Input: part model. Units: mm. Frame: model coordinates. A direction names the side the tool comes from. Round coordinates to 2 decimals unless told otherwise and drop trailing zeros. Write each loop counter-clockwise with the first axis right and the second up, starting at its lowest first coordinate (ties: lowest second). Pieces come first, ordered by that corner, then holes. Notation, with made-up numbers: (66.25, 17) -> (93.25, 17) arc R11 ccw to (93.25, 31) -> close; hole circle Ø8 at (-4.5, -9). An arc over 180 degrees is marked (long way). Write item = value, one per line.
```python
from build123d import *

# Parameters (mm, degrees)
SKETCH1_R               = 5.5
BOSS_EXTRUDE1_DEPTH     = 23
SKETCH2_R               = 4.5
BOSS_EXTRUDE2_DEPTH     = 6
SKETCH3_R               = 1.5
CUT_EXTRUDE1_DEPTH      = 6.5
CUT_EXTRUDE1_DEPTH_BACK = 6.5


with BuildPart() as part:
    # Sketch1 → Boss-Extrude1 (new body)
    with BuildSketch(Plane.XY):
        Circle(SKETCH1_R)
    extrude(amount=BOSS_EXTRUDE1_DEPTH)

    # Sketch2 → Boss-Extrude2 (add)
    with BuildSketch(Plane.XY.offset(23)):
        Circle(SKETCH2_R)
    extrude(amount=BOSS_EXTRUDE2_DEPTH)

    # Sketch3 → Cut-Extrude1 (cut, two sides)
    with BuildSketch(Plane(origin=(0, 0, 0), x_dir=(1, 0, 0), z_dir=(0, 1, 0))) as cut_extrude1_sk:
        with Locations((0, -26)):
            Circle(SKETCH3_R)
    extrude(amount=CUT_EXTRUDE1_DEPTH, mode=Mode.SUBTRACT)
    extrude(cut_extrude1_sk.sketch, amount=-CUT_EXTRUDE1_DEPTH_BACK, mode=Mode.SUBTRACT)


solid = part.part
```
1) Cut plane B-B (y = 2.5). Return the cut outline in (x, z), and give its area (3 significant figures).
Solutions:
outline = (-4.9, 0) -> (4.9, 0) -> (4.9, 23) -> (3.74, 23) -> (3.74, 29) -> (-3.74, 29) -> (-3.74, 23) -> (-4.9, 23) -> close; hole circle Ø3 at (0, 26)
area = 263 mm^2
2) Access query for faces 1 (the face through (-1.19, -5.37, 11.34)), 2 (the face through (-5, 0, 23)). Directions: +Z, -Z, +X, -X, +Y, -Y. A direction counts if a zero-diameter tool reaches every point of the face in a straight line with its end or side. Return the directions, or none.
Solutions:
face_1 = +Z, -Z
face_2 = +Z
3) Cut plane D-D (z = 6.5). Return the cut outline in (x, y).
Solutions:
outline = circle Ø11 at (0, 0)
4) First-contact query: P1, Ø3.5, axis at x = 0, z = 26, coming from the +Y side; P2, Ø5, axis at x = 0, z = 26, coming from the -Y side; P3, Ø4, axis at y = -4, z = 3, coming from the +X side. Flat tips, straight axial feed; report the tip coordinate or a pass-through.
Solutions:
P1 = 4.5
P2 = -4.5
P3 = 5.12
5) Line query: L1, parallel to Z at x = 0, y = 1.5; L2, parallel to Z at x = -0.5, y = 0; L3, parallel to X at y = 1.9, z = 26. Output: solid intervals per line, ascending. Write a range as from..to.
Solutions:
L1 = 0..24.5, 27.5..29
L2 = 0..24.59, 27.41..29
L3 = -4.08..-1.5, 1.5..4.08
6) Cut plane C-C (z = 26). Return the cut outline in (x, y).
Solutions:
outline = (-1.5, -4.24) -> (-1.5, 4.24) arc R4.5 ccw to start; (1.5, -4.24) arc R4.5 ccw to (1.5, 4.24) -> close
7) Cut plane A-A (x = 0). Return the cut outline in (y, z), and give its area (3 significant figures).
Solutions:
outline = (-5.5, 0) -> (5.5, 0) -> (5.5, 23) -> (4.5, 23) -> (4.5, 24.5) -> (-4.5, 24.5) -> (-4.5, 23) -> (-5.5, 23) -> close; (-4.5, 27.5) -> (4.5, 27.5) -> (4.5, 29) -> (-4.5, 29) -> close
area = 280 mm^2
